from build123d import *

# Parameters (mm, degrees)
BOSS_EXTRUDE1_DEPTH = 17
SKETCH2_W           = 17
SKETCH2_H           = 13
CUT_EXTRUDE1_DEPTH  = 17
CUT_EXTRUDE2_REACH  = 5
CUT_EXTRUDE3_REACH  = 5


with BuildPart() as part:
    # Sketch1 → Boss-Extrude1 (new body)
    with BuildSketch(Plane(origin=(0, 0, 0), x_dir=(1, 0, 0), z_dir=(0, 1, 0))):
        Polygon((0, 0), (20, 0), (20, 3), (3, 20), (0, 20), align=None)
    extrude(amount=BOSS_EXTRUDE1_DEPTH)

    # Sketch2 → Cut-Extrude1 (cut)
    with BuildSketch(Plane(origin=(0, 0, -20), x_dir=(-1, 0, 0), z_dir=(0, 0, -1))):
        with Locations((-11.5, 8.5)):
            Rectangle(SKETCH2_W, SKETCH2_H)
    extrude(amount=-CUT_EXTRUDE1_DEPTH, mode=Mode.SUBTRACT)

    # Sketch3 → Cut-Extrude2 (cut, up to next)
    with BuildSketch(Plane(origin=(3, 0, 0), x_dir=(0, 0, -1), z_dir=(1, 0, 0)), mode=Mode.PRIVATE) as cut_extrude2_sk1:
        with BuildLine():
            Line((9, 11.5), (11, 11.5))
            ThreePointArc((11, 11.5), (14, 8.5), (11, 5.5))
            Line((11, 5.5), (9, 5.5))
            ThreePointArc((9, 5.5), (6, 8.5), (9, 11.5))
        make_face()
    cut_extrude2_tool1 = extrude(cut_extrude2_sk1.sketch, amount=-CUT_EXTRUDE2_REACH, mode=Mode.PRIVATE) & part.part
    add(cut_extrude2_tool1.solids().sort_by_distance((3, 8.5, -10))[0], mode=Mode.SUBTRACT)

    # Sketch4 → Cut-Extrude3 (cut, up to next)
    with BuildSketch(Plane(origin=(0, 0, -3), x_dir=(-1, 0, 0), z_dir=(0, 0, -1)), mode=Mode.PRIVATE) as cut_extrude3_sk1:
        with BuildLine():
            Line((-11, 11.5), (-9, 11.5))
            ThreePointArc((-9, 11.5), (-6, 8.5), (-9, 5.5))
            Line((-9, 5.5), (-11, 5.5))
            ThreePointArc((-11, 5.5), (-14, 8.5), (-11, 11.5))
        make_face()
    cut_extrude3_tool1 = extrude(cut_extrude3_sk1.sketch, amount=-CUT_EXTRUDE3_REACH, mode=Mode.PRIVATE) & part.part
    add(cut_extrude3_tool1.solids().sort_by_distance((10, 8.5, -3))[0], mode=Mode.SUBTRACT)


solid = part.part
The listing builds one solid part. Answer for the finished solid, in the listing's coordinates (mm). A direction names the side the tool comes from. Give positions to 0.01 mm unless a question says otherwise; leave off trailing zeros. Order: outer loops, then holes, each group sorted by start corner. A loop starts at its lowest first (then second) coordinate and runs counter-clockwise, first axis right, second up. Notation, with made-up numbers: (12, -27) - (23, -27) arc R17 ccw to (23, 1) - close; hole circle Ø4 at (54, -4). An arc over 180 degrees is marked (long way). One line per item, written item: value. Start each with the question number.
1) A cutting plane is placed at B-B on x = 18.5. Give the vertices of the cut face in (y, z), then the cut area to 3 significant figures.
2) Find the intervals of material crossed by L1, parallel to Y at x = 2.25, z = -9; L2, parallel to Y at x = 13.25, z = -8.75; L3, parallel to X at y = 2.5, z = -13.75, in increasing order.
3) A cutting plane is placed at A-A on y = 8.5. Give the vertices of the cut face in (x, z), then the cut area to 3 significant figures.
4) A tool of negligible diameter and unlimited length cuts with its end or side. For faces 1 (the face through (2, 11.5, -10)), 2 (the face through (14, 11, -3)), 3 (the face through (20, 8, -1)), 4 (the face through (10, 5, 0)), 5 (the face through (6, 8.6, -1.5)), from which of +Z, -Z, +X, -X, +Y, -Y can it reach the whole face along a straight path? Write none if from no direction.
5) A cutting plane is placed at D-D on z = -7. Give the vertices of the cut face in (x, y).
6) The mould has two halves that part along Y. Classify faces 6 (the face through (10, 5.5, -2)), 7 (the face through (8, 17, -8)), 8 (the face through (12, 16, -11)): released by +Y, released by -Y, zero draft, split by the parting line, or undercut.
7) A cutting plane is placed at C-C on z = -14.75. Give the vertices of the cut face in (x, y).
8) Given pin 1 Ø2 at (y, z) = (4, -12.5) entering from +X; pin 2 Ø2 at (x, y) = (14.5, 8) entering from -Z, each flat-ended and moving along its own axis, determine where each tip first touches the part or whether it passes through.
Answer sheet:
1. outline: (0, -4.5) - (2, -4.5) - (2, -3) - (15, -3) - (15, -4.5) - (17, -4.5) - (17, 0) - (0, 0) - close
1. area: 57.0 mm2
2. L1: y = 0 to 5.5, 11.5 to 17
2. L2: y = 0 to 2, 15 to 17
2. L3: x = 0 to 3
3. outline: (0, -20) - (3, -20) - (3, -14) - (0, -14) - close; (0, -6) - (3, -6) - (3, -3) - (6, -3) - (6, 0) - (0, 0) - close; (14, -3) - (20, -3) - (20, 0) - (14, 0) - close
3. area: 63.0 mm2
4. face 1: +X, -X
4. face 2: -Z, +X
4. face 3: +Z, -Z, +X, +Y, -Y
4. face 4: +Z, +X, -X, +Y, -Y
4. face 5: +Z, -Z
5. outline: (0, 0) - (16, 0) - (16, 2) - (3, 2) - (3, 6.26) - (0, 6.26) - close; (0, 10.74) - (3, 10.74) - (3, 15) - (16, 15) - (16, 17) - (0, 17) - close
6. face 6: undercut
6. face 7: released by +Y
6. face 8: zero draft
7. outline: (0, 0) - (8.25, 0) - (8.25, 2) - (3, 2) - (3, 15) - (8.25, 15) - (8.25, 17) - (0, 17) - close
8. pin 1: stops at x = 3
8. pin 2: stops at z = -3
